from build123d import *

# Parameters (mm, degrees)
F0_W     = 67.1
F0_H     = 138.3
F1_DEPTH = 10
F2_R     = 5
F3_T     = -2.5
F4_W     = 31.3336290419
F4_H     = 11.3688334823
F5_DEPTH = 25


with BuildPart() as f1:
    # F0 (on Front) → F1 (new body, symmetric)
    with BuildSketch(Plane.XZ):
        Rectangle(F0_W, F0_H)
    extrude(amount=F1_DEPTH, both=True)

    # F2
    f2_edges = [f1.edges().sort_by_distance(p)[0] for p in [
        (-33.55, 0, 69.15),
        (33.55, 0, 69.15),
        (33.55, 0, -69.15),
        (-33.55, 0, -69.15),
    ]]
    fillet(f2_edges, radius=F2_R)

    # F3
    f3_openings = [f1.faces().sort_by_distance(p)[0] for p in [
        (0, -10, 0),
    ]]
    offset(amount=F3_T, openings=f3_openings)

    # F4 (on Front) → F5 (cut)
    with BuildSketch(Plane.XZ):
        with Locations((11.5074831992, 59.4784356654)):
            Rectangle(F4_W, F4_H)
    extrude(amount=-F5_DEPTH, mode=Mode.SUBTRACT)


solid = f1.part
Geometry: final body of the model. Coordinates: model frame, mm. A direction names the side the tool comes from. Round coordinates to 2 decimals unless told otherwise and drop trailing zeros. Loops run counter-clockwise (first coordinate to the right, second up) from the corner with the lowest first, then second, coordinate; pieces in that order, holes last. Notation, with made-up numbers: M 58,67 L 103,67 A15 cw 103,85 Z; hole C -28.5,71 d5. An arc over 180 degrees is marked long. Put each result on its own line as item: value. Start each with the question number.
(1) Section query B-B (z = -50). Return loops of the section in (x, y).
(2) Section query C-C (y = -5). Return loops of the section in (x, z), then the cut area to 3 significant figures.
(3) Section query D-D (x = -19). Return loops of the section in (y, z).
(4) Material intervals for line 1 along X through (y, z) = (0.75, -31); line 2 along Z through (x, y) = (-2.5, 0.5); line 3 along Z through (x, y) = (1, 8), sorted ascending. Write a range as [from, to].
(5) Section query A-A (x = 21.5). Return loops of the section in (y, z), then the cut area to 3 significant figures.
(6) Draft query along Z for faces 4 (the face through (33.55, 0, -1)), 5 (the face through (-32.12, -0.14, -67.65)), 6 (the face through (-32.12, 0.14, 67.65)), 7 (the face through (0, -1, 66.65)). Return one class per face: +Z half, -Z half, draft (parallel to the pull), parting line (faces both ways), or undercut.
(7) Set-up query: faces 1 (the face through (30.337, -1.373, -65.898)), 2 (the face through (11, 9, 53.794)), 3 (the face through (-32, -10, 21)). Return all of +Z, -Z, +X, -X, +Y, -Y with unobstructed straight access to the full face (end or side cutting, diameter ignored); none if empty.
(8) Contact query for a flat-ended pin moving along its axis: pin 1 Ø10 at (x, z) = (15, -6) entering from -Y. Output: stop coordinate, or through.
Findings below:
1. outline: M -33.55,-10 L -31.05,-10 L -31.05,7.5 L 31.05,7.5 L 31.05,-10 L 33.55,-10 L 33.55,10 L -33.55,10 Z
2. outline: M -33.55,-64.15 A5 ccw -28.55,-69.15 L 28.55,-69.15 A5 ccw 33.55,-64.15 L 33.55,64.15 A5 ccw 28.55,69.15 L -28.55,69.15 A5 ccw -33.55,64.15 Z; hole M -31.05,-64.15 A2.5 ccw -28.55,-66.65 L 28.55,-66.65 A2.5 ccw 31.05,-64.15 L 31.05,64.15 A2.5 ccw 28.55,66.65 L -28.55,66.65 A2.5 ccw -31.05,64.15 Z
2. area: 986 mm2
3. outline: M -10,-69.15 L 10,-69.15 L 10,69.15 L -10,69.15 L -10,66.65 L 7.5,66.65 L 7.5,-66.65 L -10,-66.65 Z
4. line 1: x = [-33.55, -31.05], [31.05, 33.55]
4. line 2: z = [-69.15, -66.65], [66.65, 69.15]
4. line 3: z = [-69.15, 53.79], [65.16, 69.15]
5. outline: M -10,-69.15 L 10,-69.15 L 10,53.79 L 7.5,53.79 L 7.5,-66.65 L -10,-66.65 Z; M -10,66.65 L 7.5,66.65 L 7.5,65.16 L 10,65.16 L 10,69.15 L -10,69.15 Z
5. area: 405 mm2
6. face 4: draft
6. face 5: -Z half
6. face 6: +Z half
6. face 7: undercut
7. face 1: -Y
7. face 2: +Y, -Y
7. face 3: +Z, -Z, +X, -X, -Y
8. pin 1: stops at y = 7.5
